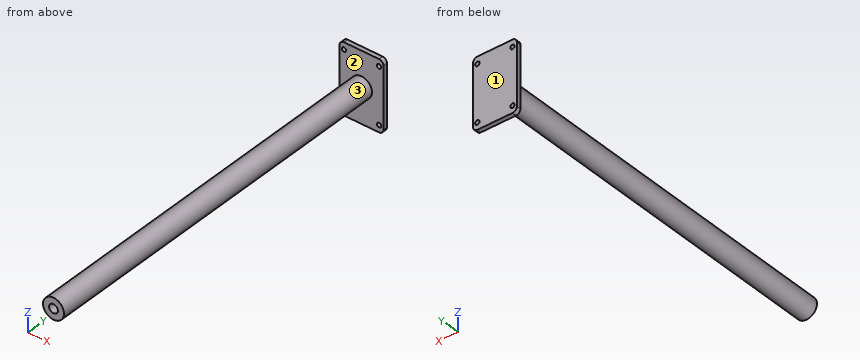
```python
from build123d import *

# Parameters (mm, degrees)
SKETCH1_R           = 12
BOSS_EXTRUDE1_DEPTH = 430
SKETCH2_R           = 2.5
BOSS_EXTRUDE2_DEPTH = 5
SKETCH3_R           = 5
CUT_EXTRUDE1_DEPTH  = 50


with BuildPart() as part:
    # Sketch1 → Boss-Extrude1 (new body)
    with BuildSketch(Plane(origin=(0, 0, 0), x_dir=(1, 0, 0), z_dir=(0, 1, 0))):
        Circle(SKETCH1_R)
    extrude(amount=-BOSS_EXTRUDE1_DEPTH)

    # Sketch2 → Boss-Extrude2 (add)
    with BuildSketch(Plane(origin=(0, 0, 0), x_dir=(1, 0, 0), z_dir=(0, 1, 0))):
        with BuildLine():
            Line((-20, 40), (20, 40))
            ThreePointArc((20, 40), (23.535533906, 38.535533906), (25, 35))
            Line((25, 35), (25, -35))
            ThreePointArc((25, -35), (23.535533906, -38.535533906), (20, -40))
            Line((20, -40), (-20, -40))
            ThreePointArc((-20, -40), (-23.535533906, -38.535533906), (-25, -35))
            Line((-25, -35), (-25, 35))
            ThreePointArc((-25, 35), (-23.535533906, 38.535533906), (-20, 40))
        make_face()
        with Locations((-20, 32)):
            Circle(SKETCH2_R, mode=Mode.SUBTRACT)
        with Locations((-20, -32)):
            Circle(SKETCH2_R, mode=Mode.SUBTRACT)
        with Locations((20, -32)):
            Circle(SKETCH2_R, mode=Mode.SUBTRACT)
        with Locations((20, 32)):
            Circle(SKETCH2_R, mode=Mode.SUBTRACT)
    extrude(amount=BOSS_EXTRUDE2_DEPTH)

    # Sketch3 → Cut-Extrude1 (cut)
    with BuildSketch(Plane.XZ.offset(430)):
        Circle(SKETCH3_R)
    extrude(amount=-CUT_EXTRUDE1_DEPTH, mode=Mode.SUBTRACT)


solid = part.part
```
Model file for the job. Use its own axes, mm. Face numbers are marked on the shaded views. Give positions to 0.01 mm unless a question says otherwise; leave off trailing zeros. Write each loop counter-clockwise with the first axis right and the second up, starting at its lowest first coordinate (ties: lowest second). Pieces come first, ordered by that corner, then holes. Notation, with made-up numbers: (10, 73.5) - (19, 73.5) arc R28 cw to (19, 108.5) - close; hole circle Ø10 at (-12, 28.5). An arc over 180 degrees is marked (long way). One line per question, with ' | ' between items. Start each with the question number.
(1) Wall check: line 1 along Z through (x, y) = (20, 2); line 2 along X through (y, z) = (2.1, 32); line 3 along Z through (x, y) = (0, -402.5). Give the ranges that are in metal, low to high. Write a range as from..to.
(2) Slice it at A-A on z = 0. Write the cut outline in (x, y).
(3) Slice it at B-B on y = -187. Write the cut outline in (x, z).
(4) Pin check, flat tips, straight feed: P1, Ø12, axis at x = -16.5, z = 20, coming from the -Y side; P2, Ø12, axis at y = -321.5, z = -12, coming from the +X side; P3, Ø8, axis at x = -4, y = -168.5, coming from the +Z side. Stop position of each tip, or through.
(5) Two-plate mould, pull along Y, no slides. Class the marked faces 1, 2 and 3: +Y half, -Y half, draft (parallel to the pull), parting line (faces both ways), or undercut.
Results below:
1) line 1: -40..-34.5, -29.5..29.5, 34.5..40 | line 2: -25..-22.5, -17.5..17.5, 22.5..25 | line 3: -12..-5, 5..12
2) outline: (-25, 0) - (-12, 0) - (-12, -430) - (-5, -430) - (-5, -380) - (5, -380) - (5, -430) - (12, -430) - (12, 0) - (25, 0) - (25, 5) - (-25, 5) - close
3) outline: circle Ø24 at (0, 0)
4) P1: y = 0 | P2: x = 10.39 | P3: z = 12
5) face 1: +Y half | face 2: -Y half | face 3: draft
